The model under review builds one solid part; all positions refer to its coordinate system, in mm. A direction names the side the tool comes from. Give positions to 0.01 mm unless a question says otherwise; leave off trailing zeros. Loops run counter-clockwise (first coordinate to the right, second up) from the corner with the lowest first, then second, coordinate; pieces in that order, holes last. Notation, with made-up numbers: M 14,86.5 L 34,86.5 A31 cw 34,122.5 Z; hole C 82,28.25 d3. An arc over 180 degrees is marked long. Write item = value, one per line. Start each with the question number.
1. Draft analysis for pull direction X (two halves, no side actions). For faces 4 (the face through (0, 3, 12.065)), 5 (the face through (11.1, 3.54, -11.05)), 6 (the face through (4.925, 1.503, 3.403)), 7 (the face through (8.961, 1.503, -10.394)), state which applies: pulls with the +X half, pulls with the -X half, needs draft (parallel to the pull), parting line crosses it, or undercut.
2. For pin 1 (1.9 mm diameter, centred on x = -8, y = 3, fed in from -Z) (3 decimals); pin 2 (3 mm diameter, centred on y = 2.5, z = -18.5, fed in from -X) (3 decimals); pin 3 (6 mm diameter, centred on x = 6.91, z = -6.91, fed in from -Y), all flat-tipped, find the tip position at first contact; note any pin that passes through.
3. Wall thickness on line 1 along Z through (x, y) = (6.75, 3.25) (3 decimals); line 2 along X through (y, z) = (5, -7) (3 decimals); line 3 along X through (y, z) = (2.5, -2.5) (3 decimals): over which ranges is each line inside the solid? List them lowest first. Write a range as from..to.
4. We need section B-B on x = -5.5. Count the separate pieces of the cut face and the enclosed holes in it, then the cut area to 3 significant figures.
5. We need section C-C on y = 7.75. Give the boundary of the cut face in (x, z) (3 decimals), then the cut area to 3 significant figures.
6. For faces 1 (the face through (-6.985, 5, -12.7)), 2 (the face through (2.878, 2, 7)), 3 (the face through (11.05, 3.54, 11.1)), list the 3-axis set-ups (+Z, -Z, +X, -X, +Y, -Y) from which the entire face can be reached by the end or side of a thin tool; tool diameter is ignored.
7. We need section A-A on x = 2.5. Give the boundary of the cut face in (y, z) (1 decimal), then the cut area to 3 significant figures.
8. We need section D-D on z = -18. Give the boundary of the cut face in (x, y) (3 decimals), then the cut area to 3 significant figures.
Autodesk Inventor part; units mm, degrees
ref_plane "YZ Plane" through (0, 0, 0) normal (1, 0, 0) x (0, 1, 0)
ref_plane "XZ Plane" through (0, 0, 0) normal (0, 1, 0) x (-1, 0, 0)
ref_plane "XY Plane" through (0, 0, 0) normal (0, 0, 1) x (1, 0, 0)
sketch "Sketch1" plane through (0, 0, 0) normal (0, 1, 0) x (-1, 0, 0)
  line L0 (-12.065, 12.065) -> (12.065, 12.065)
  line L1 (12.065, 12.065) -> (12.065, -12.065)
  line L2 (-12.065, -12.065) -> (-12.065, 12.065)
  circle A0 centre (6.9148, -6.9148) radius 1.9304
  circle A1 centre (6.9148, 6.9148) radius 1.9304
  circle A2 centre (-6.9148, 6.9148) radius 1.9304
  circle A3 centre (-6.9148, -6.9148) radius 1.9304
  line L3 (-5.715, -12.065) -> (-5.715, -21.844)
  line L4 (-5.715, -21.844) -> (6.985, -21.844)
  line L5 (6.985, -21.844) -> (6.985, -12.065)
  line L6 (12.065, -12.065) -> (6.985, -12.065)
  line L7 (-5.715, -12.065) -> (-12.065, -12.065)
  point P0 (0, 0)
  dimension "d0" = 24.13
  dimension "d2" = 12.065
  dimension "d3" = 12.065
  dimension "d4" = 3.8608
  dimension "d5" = 6.9148
  dimension "d6" = 6.9148
  dimension "d7" = 3.8608
  dimension "d8" = 6.9148
  dimension "d9" = 6.9148
  dimension "d10" = 3.8608
  dimension "d11" = 6.9148
  dimension "d12" = 6.9148
  dimension "d13" = 3.8608
  dimension "d14" = 12.7
  dimension "d16" = 6.985
  dimension "d41" = 6.9148
  dimension "d42" = 6.9148
  dimension "d43" = 24.13
  dimension "d44" = 24.13
  dimension "d50" = 9.779
  dimension "d51" = 9.779
extrude "Shape" add sketch "Sketch1" along normal blind 6.985
sketch "Sketch2" plane through (-6.985, 0, -21.844) normal (-1, 0, 0) x (0, 0, 1)
  circle A0 centre (5.08, 3.4925) radius 4.6609 construction
  line L0 (9.779, 0) -> (0, 0)
  line L1 (0, 0) -> (0, 6.985)
  line L2 (9.7409, 3.4925) -> (7.4105, -0.544)
  line L3 (7.4105, -0.544) -> (2.7496, -0.544)
  line L4 (2.7496, -0.544) -> (0.4191, 3.4925)
  line L5 (0.4191, 3.4925) -> (2.7495, 7.529)
  line L6 (2.7495, 7.529) -> (7.4104, 7.529)
  line L7 (7.4104, 7.529) -> (9.7409, 3.4925)
  line L8 (9.779, 0) -> (9.779, 6.985)
  point P0 (21.844, 0)
  dimension "d19" = 9.3218
  dimension "d20" = 3.4925
  dimension "d52" = 4.699
extrude "NutWellSide" cut sketch "Sketch2" against normal blind 3.81
sketch "Sketch3" plane through (5.715, 0, -12.065) normal (1, 0, 0) x (0, 0, -1)
  circle A0 centre (4.699, 3.4925) radius 1.9304
  line L0 (9.779, 0) -> (9.779, 6.985)
  line L1 (0, 6.985) -> (9.779, 6.985)
  line L2 (0, 0) -> (0, 6.985)
  point P0 (-12.065, 0)
  dimension "d24" = 3.8608
  dimension "d26" = 3.4925
  dimension "d53" = 4.699
extrude "HoleClamping" cut sketch "Sketch3" against normal through all
sketch "Sketch4" plane through (0, 6.985, 0) normal (0, 1, 0) x (1, 0, 0)
  circle A0 centre (0, 0) radius 6.35
  dimension "d29" = 12.7
extrude "Boss" add sketch "Sketch4" along normal blind 2.54
sketch "Sketch5" plane through (0, 9.525, 0) normal (0, 1, 0) x (1, 0, 0)
  arc A0 (2.0472, -2.5908) -> (-2.0472, -2.5908) centre (0, 0) ccw
  line L0 (-2.0472, -2.5908) -> (2.0472, -2.5908)
  dimension "d32" = 6.604
  dimension "d33" = 2.5908
fillet "Fillet1" radius 3.3782 4 edges at (12.065, 3.4925, 12.065) (12.065, 3.4925, -12.065) (-12.065, 3.4925, 12.065) (-12.065, 3.4925, -12.065)
extrude "HoleD" cut sketch "Sketch5" against normal through all
sketch "Sketch6" plane through (0, 9.525, 0) normal (0, 1, 0) x (1, 0, 0)
  line L0 (-6.985, 21.844) -> (5.715, 21.844)
  line L1 (0.127, 0.254) -> (0.127, 21.844)
  line L2 (0.127, 21.844) -> (-0.635, 20.828)
  line L3 (-0.635, 20.828) -> (-0.635, 0.254)
  line L4 (-0.1123, -19.3229) -> (0.127, 21.844) construction
  line L5 (0.6195, -20.3205) -> (-0.635, 20.828) construction
  line L6 (-0.635, 0.254) -> (0.127, 0.254)
  point P0 (0, 0)
  dimension "d37" = 1.27
extrude "ClampingSlot" cut sketch "Sketch6" against normal through all
sketch "Sketch7" plane through (0, 0, 0) normal (0, -1, 0) x (1, 0, 0)
  circle A0 centre (-6.9148, 6.9148) radius 1.9304 construction
  circle A1 centre (-6.9148, 6.9148) radius 4.6609 construction
  line L0 (-6.9148, 2.2539) -> (-10.9513, 4.5843)
  line L1 (-10.9513, 4.5843) -> (-10.9513, 9.2452)
  line L2 (-10.9513, 9.2452) -> (-6.9148, 11.5757)
  line L3 (-6.9148, 11.5757) -> (-2.8783, 9.2452)
  line L4 (-2.8783, 9.2452) -> (-2.8783, 4.5843)
  line L5 (-2.8783, 4.5843) -> (-6.9148, 2.2539)
  circle A2 centre (-6.9148, -6.9148) radius 1.9304 construction
  circle A3 centre (-6.9148, -6.9148) radius 4.6609 construction
  circle A4 centre (6.9148, -6.9148) radius 1.9304 construction
  circle A5 centre (6.9148, -6.9148) radius 4.6609 construction
  circle A6 centre (6.9148, 6.9148) radius 1.9304 construction
  circle A7 centre (6.9148, 6.9148) radius 4.6609 construction
  line L6 (6.9148, 2.2539) -> (2.8783, 4.5843)
  line L7 (2.8783, 4.5843) -> (2.8783, 9.2452)
  line L8 (2.8783, 9.2452) -> (6.9148, 11.5757)
  line L9 (6.9148, 11.5757) -> (10.9513, 9.2452)
  line L10 (10.9513, 9.2452) -> (10.9513, 4.5843)
  line L11 (10.9513, 4.5843) -> (6.9148, 2.2539)
  line L12 (6.9148, -2.2539) -> (10.9513, -4.5843)
  line L13 (10.9513, -4.5843) -> (10.9513, -9.2452)
  line L14 (10.9513, -9.2452) -> (6.9148, -11.5757)
  line L15 (6.9148, -11.5757) -> (2.8783, -9.2452)
  line L16 (2.8783, -9.2452) -> (2.8783, -4.5843)
  line L17 (2.8783, -4.5843) -> (6.9148, -2.2539)
  line L18 (-6.9148, -2.2539) -> (-2.8783, -4.5843)
  line L19 (-2.8783, -4.5843) -> (-2.8783, -9.2452)
  line L20 (-2.8783, -9.2452) -> (-6.9148, -11.5757)
  line L21 (-6.9148, -11.5757) -> (-10.9513, -9.2452)
  line L22 (-10.9513, -9.2452) -> (-10.9513, -4.5843)
  line L23 (-10.9513, -4.5843) -> (-6.9148, -2.2539)
  point P0 (0, 0)
  dimension "d40" = 9.3218
  dimension "d45" = 9.3218
  dimension "d46" = 9.3218
  dimension "d47" = 9.3218
extrude "NutWellAttachment" cut sketch "Sketch7" against normal blind 3.048
equation "\"d7\" = d4"
equation "\"d10\" = d4"
equation "\"d13\" = d4"
equation "\"d43\" = d0"
equation "\"d44\" = d0"
properties part number "clamping hub 1_4 D nut wells"
Final values:
q1.face_4 = needs draft
q1.face_5 = pulls with the +X half
q1.face_6 = undercut
q1.face_7 = undercut
q2.pin_1 = -12.065
q2.pin_2 = -3.175
q2.pin_3 = 3.05
q3.line_1 = -12.065..-8.838, -4.991..4.991, 8.838..12.065
q3.line_2 = -12.065..-8.843, -4.986..-0.635, 0.127..4.986, 8.843..12.065
q3.line_3 = -12.065..-7.341, -6.489..-2.157, 2.157..6.489, 7.341..12.065
q4.separate_pieces = 4
q4.enclosed_holes = 0
q4.area = 134 mm²
q5.outline = M -2.047,2.591 L 2.047,2.591 A3.302 cw 0.127,-3.3 L 0.127,-6.349 A6.35 ccw long -0.635,-6.318 L -0.635,-3.24 A3.302 cw Z
q5.area = 92.1 mm²
q6.face_1 = -Z, -X, +Y, -Y
q6.face_2 = -Y
q6.face_3 = +Z, +X, +Y, -Y
q7.outline = M 0,-21.8 L 7,-21.8 L 7,-5.8 L 9.5,-5.8 L 9.5,-2.2 L 0,-2.2 Z; M 0,2.2 L 9.5,2.2 L 9.5,5.8 L 7,5.8 L 7,12.1 L 0,12.1 Z; hole C 3.5,-16.8 d3.9
q7.area = 214 mm²
q8.outline = M -3.175,0 L -0.635,0 L -0.635,2.01 L -3.175,2.01 Z; M -3.175,4.975 L -0.635,4.975 L -0.635,6.985 L -3.175,6.985 Z; M 0.127,0 L 5.715,0 L 5.715,2.01 L 0.127,2.01 Z; M 0.127,4.975 L 5.715,4.975 L 5.715,6.985 L 0.127,6.985 Z
q8.area = 32.7 mm²
